from build123d import *

# Parameters (mm, degrees)
SCHIZZO1_R                     = 6.5
ESTRUSIONE_ESTRUSIONE1_DEPTH   = 35
SCHIZZO6_R                     = 1.25
TAGLIO_ESTRUSIONE4_DEPTH       = 37.187014245
TAGLIO_ESTRUSIONE5_START       = 17.4
TAGLIO_ESTRUSIONE5_OUTLINE_R   = 6.5
TAGLIO_ESTRUSIONE5_OUTLINE_R_2 = 4
TAGLIO_ESTRUSIONE5_DEPTH       = 3.1
RIPETIZIONE_A_L1_COUNT         = 2
RIPETIZIONE_A_L1_PITCH         = 9
SCHIZZO8_R                     = 5
ESTRUSIONE_ESTRUSIONE2_DEPTH   = 2
SCHIZZO9_R                     = 1.25
TAGLIO_ESTRUSIONE6_DEPTH       = 39.124795081


# Read off the part's stored shape, not the designer's step: Taglio-Estrusione5
with BuildPart() as part:
    # Schizzo1 → Estrusione-Estrusione1 (new body)
    with BuildSketch(Plane(origin=(0, 0, 0), x_dir=(1, 0, 0), z_dir=(0, 1, 0))):
        with Locations(Location((0, 0, 0), (0, 0, 270))):
            Circle(SCHIZZO1_R)
    extrude(amount=ESTRUSIONE_ESTRUSIONE1_DEPTH)

    # Schizzo6 → Taglio-Estrusione4 (cut, through all)
    with BuildSketch(Plane.XZ):
        with Locations(Location((0, 0, 0), (0, 0, 270))):
            Circle(SCHIZZO6_R)
    extrude(amount=-TAGLIO_ESTRUSIONE4_DEPTH, mode=Mode.SUBTRACT)

    # Taglio-Estrusione5 outline → Taglio-Estrusione5 (cut)
    with BuildSketch(Plane(origin=(0, 0, 0), x_dir=(1, 0, 0), z_dir=(0, 1, 0)).offset(TAGLIO_ESTRUSIONE5_START)):
        Circle(TAGLIO_ESTRUSIONE5_OUTLINE_R)
        Circle(TAGLIO_ESTRUSIONE5_OUTLINE_R_2, mode=Mode.SUBTRACT)
    taglio_estrusione5 = extrude(amount=TAGLIO_ESTRUSIONE5_DEPTH, mode=Mode.SUBTRACT)

    # Ripetizione a L1: Taglio-Estrusione5 ×2
    with Locations(*[(0, i * RIPETIZIONE_A_L1_PITCH, 0) for i in range(1, RIPETIZIONE_A_L1_COUNT)]):
        add(taglio_estrusione5, mode=Mode.SUBTRACT)

    # Schizzo8 → Estrusione-Estrusione2 (add)
    with BuildSketch(Plane.XZ):
        with Locations(Location((0, 0, 0), (0, 0, 90))):
            Circle(SCHIZZO8_R)
    extrude(amount=ESTRUSIONE_ESTRUSIONE2_DEPTH)

    # Schizzo9 → Taglio-Estrusione6 (cut, through all)
    with BuildSketch(Plane.XZ.offset(2)):
        with Locations(Location((0, 0, 0), (0, 0, 270))):
            Circle(SCHIZZO9_R)
    extrude(amount=-TAGLIO_ESTRUSIONE6_DEPTH, mode=Mode.SUBTRACT)


solid = part.part
Work out the finished part from the listing and answer in its coordinate system (mm). A direction names the side the tool comes from. Coordinates: 2 decimals unless noted, no trailing zeros. Write each loop counter-clockwise with the first axis right and the second up, starting at its lowest first coordinate (ties: lowest second). Pieces come first, ordered by that corner, then holes.
1. The part is cut by section A-A, the plane z = 0. Write down the section's boundary in (x, y).
Results list:
outline: (-6.5, 0) - (-5, 0) - (-5, -2) - (-1.25, -2) - (-1.25, 35) - (-6.5, 35) - (-6.5, 29.5) - (-4, 29.5) - (-4, 26.4) - (-6.5, 26.4) - (-6.5, 20.5) - (-4, 20.5) - (-4, 17.4) - (-6.5, 17.4) - close; (1.25, -2) - (5, -2) - (5, 0) - (6.5, 0) - (6.5, 17.4) - (4, 17.4) - (4, 20.5) - (6.5, 20.5) - (6.5, 26.4) - (4, 26.4) - (4, 29.5) - (6.5, 29.5) - (6.5, 35) - (1.25, 35) - close
2. Consider line 1 along Y through (x, z) = (2.25, 3.5); line 2 along X through (y, z) = (5, 0); line 3 along Y through (x, z) = (-5.5, -1.75). Determine where each line is inside the solid, lowest interval first.
Results list:
line 1: y = -2 to 17.4, 20.5 to 26.4, 29.5 to 35
line 2: x = -6.5 to -1.25, 1.25 to 6.5
line 3: y = 0 to 17.4, 20.5 to 26.4, 29.5 to 35
3. For faces 5 (the cylindrical face through (4.88, -0.99, -1.08)), 6 (the flat face through (3, 20.5, -3)), 7 (the cylindrical face through (1.95, 32.21, 6.2)), determine the directions among +Z, -Z, +X, -X, +Y, -Y from which every point of the face is accessible in a straight line to the end or side of a thin tool.
Results list:
face 5: -Y
face 6: none
face 7: +Y, -Y
4. A flat-ended cylindrical pin translates along its axis: pin 1 (4 mm diameter, centred on x = -3, y = 28.5, fed in from +Z). Find the tip coordinate at first contact, or state that the pin passes through.
Results list:
pin 1: stops at z = 6.38
5. For a pull along Y with two mould halves and no side action, classify faces 1 (the flat face through (3, 17.4, -3)), 2 (the flat face through (0.1, 35, 1.4)), 3 (the flat face through (-5, 0, 2)), 4 (the cylindrical face through (-1.22, 16.24, 0.27)) as +Y half, -Y half, draft (parallel to the pull), parting line (faces both ways), or undercut.
Results list:
face 1: undercut
face 2: +Y half
face 3: -Y half
face 4: draft
6. The part is cut by section D-D, the plane y = 30.5. Write down the section's boundary in (x, z), and give its area (3 significant figures).
Results list:
outline: circle Ø13 at (0, 0); hole circle Ø2.5 at (0, 0)
area: 128 mm2
7. The part is cut by section B-B, the plane x = 0. Write down the section's boundary in (y, z), and give its area (4 significant figures).
Results list:
outline: (-2, -5) - (0, -5) - (0, -6.5) - (17.4, -6.5) - (17.4, -4) - (20.5, -4) - (20.5, -6.5) - (26.4, -6.5) - (26.4, -4) - (29.5, -4) - (29.5, -6.5) - (35, -6.5) - (35, -1.25) - (-2, -1.25) - close; (-2, 1.25) - (35, 1.25) - (35, 6.5) - (29.5, 6.5) - (29.5, 4) - (26.4, 4) - (26.4, 6.5) - (20.5, 6.5) - (20.5, 4) - (17.4, 4) - (17.4, 6.5) - (0, 6.5) - (0, 5) - (-2, 5) - close
area: 351.5 mm2
8. The part is cut by section C-C, the plane z = 5.5. Write down the section's boundary in (x, y), and give its area (3 significant figures).
Results list:
outline: (-3.46, 0) - (3.46, 0) - (3.46, 17.4) - (-3.46, 17.4) - close; (-3.46, 20.5) - (3.46, 20.5) - (3.46, 26.4) - (-3.46, 26.4) - close; (-3.46, 29.5) - (3.46, 29.5) - (3.46, 35) - (-3.46, 35) - close
area: 200 mm2
